Work out the finished part from the listing and answer in its coordinate system (mm). A direction names the side the tool comes from. Coordinates: 2 decimals unless noted, no trailing zeros. Loops run counter-clockwise (first coordinate to the right, second up) from the corner with the lowest first, then second, coordinate; pieces in that order, holes last. Notation, with made-up numbers: (0, 38.5) - (21, 38.5) arc R9 ccw to (21, 42.5) - close; hole circle Ø10 at (10, 24.5). An arc over 180 degrees is marked (long way). Write each question's results on one line, items separated by ' | '. Start each with the question number.
1. Find the intervals of material crossed by line 1 along X through (y, z) = (0, 0); line 2 along Z through (x, y) = (24.5, 7.5); line 3 along X through (y, z) = (0, -1.75), in increasing order. Write a range as [from, to].
2. Which of the six approach directions +Z, -Z, +X, -X, +Y, -Y give full straight-line access (tool end or side, diameter ignored) to faces 1 (the cylindrical face through (60.294, 3.494, 5.481)), 2 (the flat face through (28.49, -24.98, 9.48)), 3 (the flat face through (-18, 0, 8.5))?
3. Determine the mould class of faces 4 (the cylindrical face through (69.524, 0.92, 0.091)), 5 (the flat face through (-11.4, 13.1, 4.4)), 6 (the flat face through (-57.414, -7.03, 4.444)) for opening direction Y: released by +Y, released by -Y, zero draft, split by the parting line, or undercut.
4. A cutting plane is placed at D-D on z = 4. Determine the outline of the cut face in (x, y).
5. Each of these flat-tipped pins is pushed along its axis until it touches: P1, Ø6, axis at x = 12, y = 8.5, coming from the -Z side; P2, Ø11, axis at y = -14.5, z = -3.5, coming from the -X side; P3, Ø6, axis at x = 8.5, z = 8, coming from the -Y side. Where does it stop, or does it pass through?
6. A cutting plane is placed at A-A on z = -2.25. Determine the outline of the cut face in (x, y), then the cut area to 3 significant figures.
7. A cutting plane is placed at B-B on x = -41. Determine the outline of the cut face in (y, z), then the cut area to 3 significant figures.
8. A cutting plane is placed at C-C on y = 11.5. Determine the outline of the cut face in (x, z).
from build123d import *

# Parameters (mm, degrees)
F1_DEPTH     = 12.5
F2_DEPTH     = 8.5
F3_SIZE      = 8
F4_T1_DEPTH  = 6.3508529611
F4_T3_DEPTH  = 6.3508529611
F4_T5_DEPTH  = 6.3508529611
F4_T7_DEPTH  = 6.3508529611
F4_T9_DEPTH  = 6.3508529611
F4_T11_DEPTH = 6.3508529611
F4_T13_DEPTH = 6.3508529611
F4_T15_DEPTH = 6.3508529611
F4_T17_DEPTH = 50.7168298797
F4_T19_DEPTH = 47.7168298797
F4_T21_DEPTH = 82.7168298797
F4_T26_DEPTH = 82.7168298797
F4_T31_DEPTH = 82.7168298797
F4_T36_DEPTH = 82.7168298797
F4_T41_DEPTH = 82.7168298797
F4_T46_DEPTH = 82.7168298797
F4_T51_DEPTH = 82.7168298797
F5_R         = 6.5
F6_DEPTH     = 26.9
F7_R         = 3.0614301368
F8_DEPTH     = 6.5


# Not quite as in the source:
# - a fillet or chamfer that OpenCascade refuses, or shapes differently, is made with other operations: its cross-section is extruded or revolved along the edge and cut away or added


with BuildPart() as f1:
    # F0 (on Top) → F1 (new body, symmetric)
    with BuildSketch(Plane.XY):
        Polygon((25.0318072736, -28.5), (47.0318072736, -28.5), (47.0318072736, 0), (47.0318072736, 28.5), (25.0318072736, 28.5), (25.0318072736, 17), (25.0318072736, -17), align=None)
    extrude(amount=F1_DEPTH, both=True)

    # F0 (on Top) → F2 (join, symmetric)
    with BuildSketch(Plane.XY):
        Polygon((-49.9681927264, -17), (25.0318072736, -17), (25.0318072736, 17), (-49.9681927264, 17), (-74.4579061866, 0), align=None)
    extrude(amount=F2_DEPTH, both=True)

    # F3
    f3_edges = [f1.edges().sort_by_distance(p)[0] for p in [
        (-12.468193, 17, -8.5),
        (-12.468193, -17, -8.5),
        (-62.213049, -8.5, -8.5),
        (-12.468193, -17, 8.5),
        (-12.468193, 17, 8.5),
        (-62.213049, -8.5, 8.5),
        (-62.213049, 8.5, 8.5),
        (-62.213049, 8.5, -8.5),
    ]]
    chamfer(f3_edges, length=F3_SIZE)

    # F4: chamfer of 5 on 12 edges, made by hand

    # F4_s2 → F4_t1 (cut)
    with BuildSketch(Plane(origin=(-1.9893975755, 1.9893975755, -1.9893975755), x_dir=(-0.7071067812, -0.7071067812, 0), z_dir=(-0.5773502692, 0.5773502692, -0.5773502692))):
        Polygon((-34.3171700264, -6.7490820577), (-37.8527039324, -12.8728064147), (-41.3882378383, -6.7490820577), align=None)
    extrude(amount=F4_T1_DEPTH, mode=Mode.SUBTRACT)

    # F4_s4 → F4_t3 (cut)
    with BuildSketch(Plane(origin=(-1.9893975755, -1.9893975755, -1.9893975755), x_dir=(0.7071067812, -0.7071067812, 0), z_dir=(-0.5773502692, -0.5773502692, -0.5773502692))):
        Polygon((34.3171700264, -6.7490820577), (41.3882378383, -6.7490820577), (37.8527039324, -12.8728064147), align=None)
    extrude(amount=F4_T3_DEPTH, mode=Mode.SUBTRACT)

    # F4_s6 → F4_t5 (cut)
    with BuildSketch(Plane(origin=(-1.9893975755, -1.9893975755, 1.9893975755), x_dir=(0.7071067812, -0.7071067812, 0), z_dir=(-0.5773502692, -0.5773502692, 0.5773502692))):
        Polygon((34.3171700264, 6.7490820577), (41.3882378383, 6.7490820577), (37.8527039324, 12.8728064147), align=None)
    extrude(amount=F4_T5_DEPTH, mode=Mode.SUBTRACT)

    # F4_s8 → F4_t7 (cut)
    with BuildSketch(Plane(origin=(-1.9893975755, 1.9893975755, 1.9893975755), x_dir=(-0.7071067812, -0.7071067812, 0), z_dir=(-0.5773502692, 0.5773502692, 0.5773502692))):
        Polygon((-34.3171700264, 6.7490820577), (-37.8527039324, 12.8728064147), (-41.3882378383, 6.7490820577), align=None)
    extrude(amount=F4_T7_DEPTH, mode=Mode.SUBTRACT)

    # F4_s10 → F4_t9 (cut)
    with BuildSketch(Plane(origin=(26.0106024245, 26.0106024245, -26.0106024245), x_dir=(-0.7071067812, 0.7071067812, 0), z_dir=(0.5773502692, 0.5773502692, -0.5773502692))):
        Polygon((-16.6395004968, 22.6707653858), (-13.1039665908, 16.5470410289), (-9.5684326849, 22.6707653858), align=None)
    extrude(amount=F4_T9_DEPTH, mode=Mode.SUBTRACT)

    # F4_s12 → F4_t11 (cut)
    with BuildSketch(Plane(origin=(26.0106024245, 26.0106024245, 26.0106024245), x_dir=(-0.7071067812, 0.7071067812, 0), z_dir=(0.5773502692, 0.5773502692, 0.5773502692))):
        Polygon((-13.1039665908, -16.5470410289), (-16.6395004968, -22.6707653858), (-9.5684326849, -22.6707653858), align=None)
    extrude(amount=F4_T11_DEPTH, mode=Mode.SUBTRACT)

    # F4_s14 → F4_t13 (cut)
    with BuildSketch(Plane(origin=(26.0106024245, -26.0106024245, -26.0106024245), x_dir=(0.7071067812, 0.7071067812, 0), z_dir=(0.5773502692, -0.5773502692, -0.5773502692))):
        Polygon((16.6395004968, 22.6707653858), (9.5684326849, 22.6707653858), (13.1039665908, 16.5470410289), align=None)
    extrude(amount=F4_T13_DEPTH, mode=Mode.SUBTRACT)

    # F4_s16 → F4_t15 (cut)
    with BuildSketch(Plane(origin=(26.0106024245, -26.0106024245, 26.0106024245), x_dir=(0.7071067812, 0.7071067812, 0), z_dir=(0.5773502692, -0.5773502692, 0.5773502692))):
        Polygon((9.5684326849, -22.6707653858), (13.1039665908, -16.5470410289), (16.6395004968, -22.6707653858), align=None)
    extrude(amount=F4_T15_DEPTH, mode=Mode.SUBTRACT)

    # F4_s18 → F4_t17 (cut)
    with BuildSketch(Plane.XY.offset(-25.3584149398)):
        Polygon((25.0318072736, -23.5), (30.0318072736, -28.5), (25.0318072736, -28.5), align=None)
        Polygon((25.0318072736, 23.5), (30.0318072736, 28.5), (25.0318072736, 28.5), align=None)
        Polygon((42.0318072736, 28.5), (47.0318072736, 23.5), (47.0318072736, 28.5), align=None)
        Polygon((42.0318072736, -28.5), (47.0318072736, -23.5), (47.0318072736, -28.5), align=None)
    extrude(amount=F4_T17_DEPTH, mode=Mode.SUBTRACT)

    # F4_s20 → F4_t19 (cut)
    with BuildSketch(Plane.YZ.offset(12.1733923338)):
        Polygon((23.5, -12.5), (28.5, -7.5), (28.5, -12.5), align=None)
        Polygon((23.5, 12.5), (28.5, 7.5), (28.5, 12.5), align=None)
        Polygon((-28.5, -7.5), (-23.5, -12.5), (-28.5, -12.5), align=None)
        Polygon((-28.5, 7.5), (-23.5, 12.5), (-28.5, 12.5), align=None)
    extrude(amount=F4_T19_DEPTH, mode=Mode.SUBTRACT)

    # F4_s22 → F4_t21 (cut)
    with BuildSketch(Plane.XZ.offset(-41.3584149398)):
        Polygon((42.0318072736, 12.5), (47.0318072736, 7.5), (47.0318072736, 12.5), align=None)
        Polygon((42.0318072736, -12.5), (47.0318072736, -7.5), (47.0318072736, -12.5), align=None)
    extrude(amount=F4_T21_DEPTH, mode=Mode.SUBTRACT)


with BuildPart() as f4_tool24:
    # F4_s25 → F4_t26 (new body)
    with BuildSketch(Plane.XZ.offset(-41.3584149398)):
        Polygon((25.0318072736, -7.5), (30.0318072736, -12.5), (25.0318072736, -12.5), align=None)
    extrude(amount=F4_T26_DEPTH)

    split(bisect_by=Plane(origin=(0, 8.75, -8.75), x_dir=(1, 0, 0), z_dir=(0, 0.7071067812, -0.7071067812)), keep=Keep.TOP)


with BuildPart() as f1_1:
    add(f1.part)

    # F4_t23: cut F4_tool24
    add(f4_tool24.part, mode=Mode.SUBTRACT)


with BuildPart() as f4_tool29:
    # F4_s30 → F4_t31 (new body)
    with BuildSketch(Plane.XZ.offset(-41.3584149398)):
        Polygon((25.0318072736, -7.5), (30.0318072736, -12.5), (25.0318072736, -12.5), align=None)
    extrude(amount=F4_T31_DEPTH)

    split(bisect_by=Plane.XY.offset(-8.5), keep=Keep.BOTTOM)


with BuildPart() as f1_2:
    add(f1_1.part)

    # F4_t28: cut F4_tool29
    add(f4_tool29.part, mode=Mode.SUBTRACT)


with BuildPart() as f4_tool34:
    # F4_s35 → F4_t36 (new body)
    with BuildSketch(Plane.XZ.offset(-41.3584149398)):
        Polygon((25.0318072736, -7.5), (30.0318072736, -12.5), (25.0318072736, -12.5), align=None)
    extrude(amount=F4_T36_DEPTH)

    split(bisect_by=Plane(origin=(0, -8.75, -8.75), x_dir=(1, 0, 0), z_dir=(0, -0.7071067812, -0.7071067812)), keep=Keep.TOP)


with BuildPart() as f1_3:
    add(f1_2.part)

    # F4_t33: cut F4_tool34
    add(f4_tool34.part, mode=Mode.SUBTRACT)


with BuildPart() as f4_tool39:
    # F4_s40 → F4_t41 (new body)
    with BuildSketch(Plane.XZ.offset(41.3584149398)):
        Polygon((25.0318072736, 7.5), (30.0318072736, 12.5), (25.0318072736, 12.5), align=None)
    extrude(amount=-F4_T41_DEPTH)

    split(bisect_by=Plane(origin=(0, -8.75, 8.75), x_dir=(1, 0, 0), z_dir=(0, -0.7071067812, 0.7071067812)), keep=Keep.TOP)


with BuildPart() as f1_4:
    add(f1_3.part)

    # F4_t38: cut F4_tool39
    add(f4_tool39.part, mode=Mode.SUBTRACT)


with BuildPart() as f4_tool44:
    # F4_s45 → F4_t46 (new body)
    with BuildSketch(Plane.XZ.offset(41.3584149398)):
        Polygon((25.0318072736, 7.5), (30.0318072736, 12.5), (25.0318072736, 12.5), align=None)
    extrude(amount=-F4_T46_DEPTH)

    split(bisect_by=Plane.XY.offset(8.5), keep=Keep.TOP)


with BuildPart() as f1_5:
    add(f1_4.part)

    # F4_t43: cut F4_tool44
    add(f4_tool44.part, mode=Mode.SUBTRACT)


with BuildPart() as f4_tool49:
    # F4_s50 → F4_t51 (new body)
    with BuildSketch(Plane.XZ.offset(41.3584149398)):
        Polygon((25.0318072736, 7.5), (30.0318072736, 12.5), (25.0318072736, 12.5), align=None)
    extrude(amount=-F4_T51_DEPTH)

    split(bisect_by=Plane(origin=(0, 8.75, 8.75), x_dir=(1, 0, 0), z_dir=(0, 0.7071067812, 0.7071067812)), keep=Keep.TOP)


with BuildPart() as f1_6:
    add(f1_5.part)

    # F4_t48: cut F4_tool49
    add(f4_tool49.part, mode=Mode.SUBTRACT)

    # F5 (on face) → F6 (join)
    with BuildSketch(Plane.YZ.offset(47.0318072736)):
        Circle(F5_R)
    extrude(amount=F6_DEPTH)

    # F7 (on Top) → F8 (cut, symmetric)
    with BuildSketch(Plane.XY):
        with Locations((66.6042044759, 0)):
            Circle(F7_R)
    extrude(amount=F8_DEPTH, both=True, mode=Mode.SUBTRACT)


solid = f1_6.part
Values:
1) line 1: [-74.46, 63.54], [69.67, 73.93] | line 2: [-8.5, 8.5] | line 3: [-72.27, 63.54], [69.67, 73.93]
2) face 1: +X | face 2: +Z, -X, -Y | face 3: +Z, -X, +Y, -Y
3) face 4: undercut | face 5: released by +Y | face 6: released by -Y
4) outline: (-68.32, 0) - (-48.87, -13.5) - (25.03, -13.5) - (25.03, -23.5) - (30.03, -28.5) - (42.03, -28.5) - (47.03, -23.5) - (47.03, -5.12) - (73.93, -5.12) - (73.93, 5.12) - (47.03, 5.12) - (47.03, 23.5) - (42.03, 28.5) - (30.03, 28.5) - (25.03, 23.5) - (25.03, 13.5) - (-48.87, 13.5) - close; hole circle Ø6.12 at (66.6, 0)
5) P1: z = -8.5 | P2: x = -60.21 | P3: y = -12.5
6) outline: (-71.39, 0) - (-49.42, -15.25) - (25.03, -15.25) - (25.03, -23.5) - (30.03, -28.5) - (42.03, -28.5) - (47.03, -23.5) - (47.03, -6.1) - (73.93, -6.1) - (73.93, 6.1) - (47.03, 6.1) - (47.03, 23.5) - (42.03, 28.5) - (30.03, 28.5) - (25.03, 23.5) - (25.03, 15.25) - (-49.42, 15.25) - close; hole circle Ø6.12 at (66.6, 0) | area: 4,110 mm^2
7) outline: (-17, -0.5) - (-9, -8.5) - (9, -8.5) - (17, -0.5) - (17, 0.5) - (9, 8.5) - (-9, 8.5) - (-17, 0.5) - close | area: 450 mm^2
8) outline: (-57.89, -0.5) - (-48.25, -6) - (25.03, -6) - (25.03, -7.5) - (30.03, -12.5) - (42.03, -12.5) - (47.03, -7.5) - (47.03, 7.5) - (42.03, 12.5) - (30.03, 12.5) - (25.03, 7.5) - (25.03, 6) - (-48.25, 6) - (-57.89, 0.5) - close
